Check sheet for the modelled part. Datum: model origin and axes. Units: mm. A direction names the side the tool comes from. Round coordinates to 2 decimals unless told otherwise and drop trailing zeros. Order: outer loops, then holes, each group sorted by start corner. A loop starts at its lowest first (then second) coordinate and runs counter-clockwise, first axis right, second up.
from build123d import *

# Parameters (mm, degrees)
SKETCH1_W               = 60
SKETCH1_H               = 60
BOSS_EXTRUDE1_DEPTH     = 100
SKETCH4_R               = 2.5
BOSS_EXTRUDE2_DEPTH     = 2.5
CUT_EXTRUDE1_DEPTH      = 169.893457541
CUT_EXTRUDE1_DEPTH_BACK = 169.893457541
SKETCH5_R               = 2.5
SKETCH6_W               = 60
SKETCH6_H               = 60
CUT_EXTRUDE2_DEPTH      = 2.5
CHAMFER1_SIZE           = 2
CHAMFER2_SIZE           = 5
SKETCH7_W               = 55
SKETCH7_H               = 55
CUT_EXTRUDE3_DEPTH      = 35
SKETCH8_W               = 46
SKETCH8_H               = 55
CUT_EXTRUDE4_DEPTH      = 35
CUT_EXTRUDE5_DEPTH      = 46
SKETCH10_W              = 5
SKETCH10_H              = 60
CUT_EXTRUDE6_DEPTH      = 30
CHAMFER3_SIZE           = 3


with BuildPart() as part:
    # Sketch1 → Boss-Extrude1 (new body)
    with BuildSketch(Plane(origin=(0, 0, 0), x_dir=(1, 0, 0), z_dir=(0, 1, 0))):
        Rectangle(SKETCH1_W, SKETCH1_H)
    extrude(amount=BOSS_EXTRUDE1_DEPTH)

    # Sketch4 → Boss-Extrude2 (add)
    with BuildSketch(Plane(origin=(0, 0, -30), x_dir=(-1, 0, 0), z_dir=(0, 0, -1))):
        with BuildLine():
            Line((-30, 100), (30, 100))
            Line((30, 100), (30, 125))
            ThreePointArc((30, 125), (0, 155), (-30, 125))
            Line((-30, 125), (-30, 100))
        make_face()
        with Locations((0, 125)):
            Circle(SKETCH4_R, mode=Mode.SUBTRACT)
    boss_extrude2 = extrude(amount=-BOSS_EXTRUDE2_DEPTH)

    # Mirror2: Boss-Extrude2 across plane
    add(boss_extrude2.mirror(Plane.XY))

    # Sketch5 → Cut-Extrude1 (cut, two sides: drawn at the far end of the back side and taken through both)
    with BuildSketch(Plane.ZY.offset(-30).offset(-CUT_EXTRUDE1_DEPTH_BACK)):
        with BuildLine():
            Line((-30, 0), (2.9e-08, 0))
            ThreePointArc((2.9e-08, 0), (-21.213203425, 8.786796554), (-30, 30))
            Line((-30, 30), (-30, 0))
        make_face()
        with BuildLine():
            Line((30, 0), (30, 30))
            ThreePointArc((30, 30), (21.213203446, 8.786796575), (2.9e-08, 0))
            Line((2.9e-08, 0), (30, 0))
        make_face()
        with Locations((0, 30)):
            Circle(SKETCH5_R)
    extrude(amount=CUT_EXTRUDE1_DEPTH + CUT_EXTRUDE1_DEPTH_BACK, mode=Mode.SUBTRACT)

    # Sketch6 → Cut-Extrude2 (cut)
    with BuildSketch(Plane(origin=(30, 0, 0), x_dir=(0, 0, -1), z_dir=(1, 0, 0))):
        with Locations((0, 30)):
            Rectangle(SKETCH6_W, SKETCH6_H)
    cut_extrude2 = extrude(amount=-CUT_EXTRUDE2_DEPTH, mode=Mode.SUBTRACT)

    # Mirror3: Cut-Extrude2 across plane
    add(cut_extrude2.mirror(Plane(origin=(0, 0, 0), x_dir=(0, 0, 1), z_dir=(1, 0, 0))), mode=Mode.SUBTRACT)

    # Chamfer1
    chamfer1_edges = [part.edges().sort_by_distance(p)[0] for p in [
        (-30, 100, 0),
        (0, 155, -30),
        (30, 100, 0),
        (0, 155, 30),
        (30, 92.5, 30),
        (-30, 92.5, 30),
        (-30, 92.5, -30),
        (30, 92.5, -30),
    ]]
    chamfer(chamfer1_edges, length=CHAMFER1_SIZE)

    # Chamfer2
    # the kernel refuses this chamfer: 5 mm, written as the material it takes off along each edge
    with BuildSketch(Plane(origin=(30, 60, 40.85841494), x_dir=(0.027495876610586282, 0.9996219169112968, 0), z_dir=(0, 0, -1))) as chamfer2_piece_1_section:
        Polygon((CHAMFER2_SIZE * 0.999621916911, -CHAMFER2_SIZE * 0.0274958766106), (-CHAMFER2_SIZE * 0.0274958766106, -CHAMFER2_SIZE * 0.999621916911), (0, 0), align=None)
    chamfer2_piece_1 = extrude(amount=81.71682988, mode=Mode.PRIVATE)
    chamfer2_piece_1 = split(chamfer2_piece_1, bisect_by=Plane(origin=(27.5, 61.967005421, 0), z_dir=(1, 0, 0)), keep=Keep.TOP, mode=Mode.PRIVATE)
    add(chamfer2_piece_1, mode=Mode.SUBTRACT)
    with BuildSketch(Plane(origin=(-30, 60, 40.85841494), x_dir=(-0.027495876610586282, 0.9996219169112968, 0), z_dir=(0, 0, -1))) as chamfer2_piece_2_section:
        Polygon((CHAMFER2_SIZE * 0.999621916911, CHAMFER2_SIZE * 0.0274958766106), (-CHAMFER2_SIZE * 0.0274958766106, CHAMFER2_SIZE * 0.999621916911), (0, 0), align=None)
    chamfer2_piece_2 = extrude(amount=81.71682988, mode=Mode.PRIVATE)
    chamfer2_piece_2 = split(chamfer2_piece_2, bisect_by=Plane(origin=(-27.5, 61.967005421, 0), z_dir=(-1, 0, 0)), keep=Keep.TOP, mode=Mode.PRIVATE)
    add(chamfer2_piece_2, mode=Mode.SUBTRACT)

    # Sketch7 → Cut-Extrude3 (cut)
    with BuildSketch(Plane(origin=(0, 100, 0), x_dir=(1, 0, 0), z_dir=(0, 1, 0))):
        Rectangle(SKETCH7_W, SKETCH7_H)
    extrude(amount=-CUT_EXTRUDE3_DEPTH, mode=Mode.SUBTRACT)

    # Sketch8 → Cut-Extrude4 (cut)
    with BuildSketch(Plane(origin=(0, 65, 0), x_dir=(1, 0, 0), z_dir=(0, 1, 0))):
        Rectangle(SKETCH8_W, SKETCH8_H)
    extrude(amount=-CUT_EXTRUDE4_DEPTH, mode=Mode.SUBTRACT)

    # Sketch9 → Cut-Extrude5 (cut)
    with BuildSketch(Plane.ZY.offset(-23)):
        with BuildLine():
            Line((-27.5, 30), (27.5, 30))
            ThreePointArc((27.5, 30), (0, 2.5), (-27.5, 30))
        make_face()
    extrude(amount=CUT_EXTRUDE5_DEPTH, mode=Mode.SUBTRACT)

    # Sketch10 → Cut-Extrude6 (cut)
    with BuildSketch(Plane(origin=(0, 0, 0), x_dir=(1, 0, 0), z_dir=(0, 1, 0))):
        Rectangle(SKETCH10_W, SKETCH10_H)
    extrude(amount=CUT_EXTRUDE6_DEPTH, mode=Mode.SUBTRACT)

    # Chamfer3
    chamfer3_edges = [part.edges().sort_by_distance(p)[0] for p in [
        (23, 65, 0),
        (-23, 65, 0),
    ]]
    chamfer(chamfer3_edges, length=CHAMFER3_SIZE)


solid = part.part
1) Sectioned sample at D-D on y = 38. Record the cut outline in (x, z), and give its area (3 significant figures).
2) Sectioned sample at B-B on y = 89. Record the cut outline in (x, z), and give its area (3 significant figures).
3) Sectioned sample at C-C on z = 18. Record the cut outline in (x, y), and give its area (3 significant figures).
4) Set-up check for faces 5 (the face through (0, 92, 30)), 6 (the face through (-27.5, 39, 0)), 7 (the face through (-27.5, 83, 0)), 8 (the face through (27.5, 38, 0)): record each of +Z, -Z, +X, -X, +Y, -Y from which the full face is reachable in a straight line by a thin tool's end or side.
5) Sectioned sample at A-A on x = 0. Record the cut outline in (y, z), and give its area (3 significant figures).
6) Scan lines: line 1 (Z direction, x = -12.5, y = 73); line 2 (Z direction, x = -25.55, y = 30). Record each from-to range of solid material in increasing order.
7) Draft check along X on faces 1 (the face through (-0.66, 154.993, -27.754)), 2 (the face through (2.5, 2.7, 4.6)), 3 (the face through (-2.5, 2.7, 4.6)), 4 (the face through (30, 82, 0)). Enter one of: pulls with the +X half, pulls with the -X half, needs draft (parallel to the pull), parting line crosses it, or undercut.
8) Gauge pin test, flat ends, axial feed: pin 1 (18 mm diameter, centred on y = 17.5, z = -12.5, fed in from +X); pin 2 (0.8 mm diameter, centred on x = -0.5, z = 29.5, fed in from -Y); pin 3 (10 mm diameter, centred on y = 124.5, z = 23.5, fed in from +X); pin 4 (6.5 mm diameter, centred on y = 30, z = 0, fed in from -X). Record the tip position at first contact, or that the pin passes through.
Values found:
1. outline: (-27.5, -30) - (27.5, -30) - (27.5, 30) - (-27.5, 30) - close; hole (-23, -27.5) - (23, -27.5) - (23, 27.5) - (-23, 27.5) - close
1. area: 770 mm2
2. outline: (-30, -28) - (-28, -30) - (28, -30) - (30, -28) - (30, 28) - (28, 30) - (-28, 30) - (-30, 28) - close; hole (-27.5, -27.5) - (27.5, -27.5) - (27.5, 27.5) - (-27.5, 27.5) - close
2. area: 567 mm2
3. outline: (-30, 65) - (-27.5, 62.5) - (-27.5, 6) - (-2.5, 6) - (-2.5, 9.21) - (-23, 9.21) - (-23, 62) - (-26, 65) - (-27.5, 65) - (-27.5, 100) - (-28, 100) - (-30, 98) - close; (2.5, 6) - (27.5, 6) - (27.5, 62.5) - (30, 65) - (30, 98) - (28, 100) - (27.5, 100) - (27.5, 65) - (26, 65) - (23, 62) - (23, 9.21) - (2.5, 9.21) - close
3. area: 831 mm2
4. face 5: +Z, +X, -X, +Y, -Y
4. face 6: +Z, -Z, -X, -Y
4. face 7: +Y
4. face 8: +Z, -Z, +X, -Y
5. outline: (30, -30) - (122.5, -30) - (122.5, -27.5) - (30, -27.5) - close; (30, 27.5) - (122.5, 27.5) - (122.5, 30) - (30, 30) - close; (127.5, -30) - (153, -30) - (155, -28) - (155, -27.5) - (127.5, -27.5) - close; (127.5, 27.5) - (155, 27.5) - (155, 28) - (153, 30) - (127.5, 30) - close
5. area: 596 mm2
6. line 1: z = -30 to -27.5, 27.5 to 30
6. line 2: z = -30 to -2.5, 2.5 to 30
7. face 1: parting line crosses it
7. face 2: undercut
7. face 3: undercut
7. face 4: pulls with the +X half
8. pin 1: stops at x = 27.5
8. pin 2: stops at y = 30
8. pin 3: stops at x = 30
8. pin 4: stops at x = -27.5
